Autodesk Inventor part; units mm, degrees
ref_plane "YZ Plane" through (0, 0, 0) normal (1, 0, 0) x (0, 1, 0)
ref_plane "XZ Plane" through (0, 0, 0) normal (0, 1, 0) x (-1, 0, 0)
ref_plane "XY Plane" through (0, 0, 0) normal (0, 0, 1) x (1, 0, 0)
sketch "Sketch1" plane through (0, 0, 0) normal (0, 1, 0) x (-1, 0, 0)
  circle A0 centre (0, 0) radius 8.575
  dimension "d0" = 17.15
extrude "Extrusion1" add sketch "Sketch1" along normal blind 75.5
sketch "Sketch2" plane through (0, 75.5, 0) normal (0, 1, 0) x (1, 0, 0)
  circle A0 centre (0, 0) radius 8.85
  dimension "d3" = 17.7
extrude "Extrusion2" add sketch "Sketch2" against normal blind 9.6
sketch "Sketch3" plane through (0, 75.5, 0) normal (0, 1, 0) x (1, 0, 0)
  line L0 (-3.3083, -9.5957) -> (-10.4021, -7.15)
  arc A0 (-10.4021, 7.15) -> (-10.4021, -7.15) centre (-7.937, 0) ccw
  line L1 (-10.4021, 7.15) -> (-3.3083, 9.5957)
  arc A1 (3.3083, 9.5957) -> (-3.3083, 9.5957) centre (0, 0) ccw
  line L2 (3.3083, 9.5957) -> (10.4021, 7.15)
  arc A2 (10.4021, -7.15) -> (10.4021, 7.15) centre (7.937, 0) ccw
  line L3 (10.4021, -7.15) -> (3.3083, -9.5957)
  arc A3 (-3.3083, -9.5957) -> (3.3083, -9.5957) centre (0, 0) ccw
  line L4 (0, -10.15) -> (0, 10.15) construction
  line L5 (-15.5, 0) -> (15.5, 0) construction
  dimension "d6" = 20.3
  dimension "d7" = 31
  dimension "d8" = 14.3
extrude "Extrusion3" add sketch "Sketch3" against normal blind 2
sketch "Sketch4" plane through (0, 75.5, 0) normal (0, 1, 0) x (1, 0, 0)
  circle A0 centre (0, 0) radius 7.875
  dimension "d11" = 15.75
extrude "Extrusion4" cut sketch "Sketch4" against normal blind 74.5
sketch "Sketch5" plane through (0, 0, 0) normal (0, -1, 0) x (1, 0, 0)
  circle A0 centre (0, -5.075) radius 2.5
  point P0 (0, 0)
  dimension "d14" = 5
ref_plane "Work Plane1" through (0, -10, 0) normal (0, -1, 0) x (1, 0, 0)
sketch "Sketch6" plane through (0, -10, 0) normal (0, -1, 0) x (1, 0, 0)
  circle A0 centre (0, -5.075) radius 2
  point P0 (0, 0)
  dimension "d18" = 4
loft "Loft1" add profiles "Sketch5", "Sketch6"
sketch "Sketch7" plane through (0, -10, -5.075) normal (0, -1, 0) x (1, 0, 0)
  circle A0 centre (0, 0) radius 2
  circle A1 centre (0, 0) radius 1.2
  point P0 (0, 5.075)
  dimension "d24" = 0.8
extrude "Extrusion5" cut sketch "Sketch7" against normal through all contours A1
properties part number "Syringe" material "Glass"
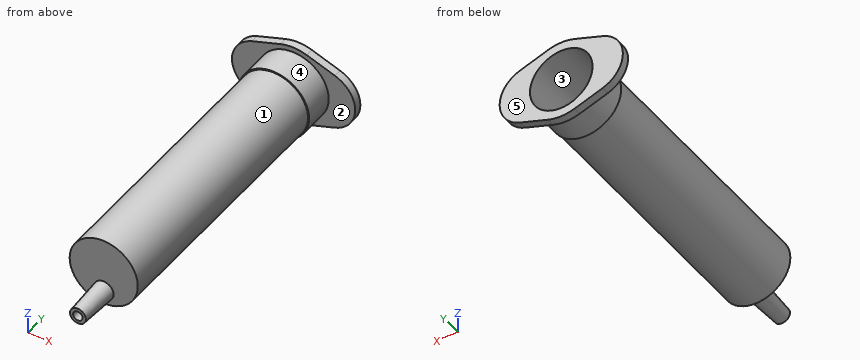
Could you check a few things on this model? Use its own coordinates, in mm. Face numbers are marked on the shaded views. A direction names the side the tool comes from. Round coordinates to 2 decimals unless told otherwise and drop trailing zeros. Loops run counter-clockwise (first coordinate to the right, second up) from the corner with the lowest first, then second, coordinate; pieces in that order, holes last. Notation, with made-up numbers: (18, 81.25) - (40, 81.25) arc R24 ccw to (40, 119.25) - close; hole circle Ø1 at (-20, 80). An arc over 180 degrees is marked (long way). Write item = value, one per line.
1) I need wall thicknesses on line 1 along X through (y, z) = (18, -0.25); line 2 along Z through (x, y) = (0, 45) (3 decimals); line 3 along Y through (x, z) = (0, -8.5). Which ranges of each line are inside material? Lowest first, please. Write a range as from..to.
Computed:
line_1 = -8.57..-7.87, 7.87..8.57
line_2 = -8.575..-7.875, 7.875..8.575
line_3 = 0..75.5
2) If we mould it in two halves opening along Z, with no side actions, what happens to the marked faces 1, 2 and 3? For each: pulls with the +Z half, pulls with the -Z half, needs draft (parallel to the pull), parting line crosses it, or undercut.
Computed:
face_1 = parting line crosses it
face_2 = needs draft
face_3 = undercut
3) I'm going to push flat-ended pins straight in: P1, Ø8, axis at x = 11, z = 4.5, coming from the -Y side; P2, Ø2, axis at y = 15, z = 6, coming from the -X side; P3, Ø9.5, axis at x = 0, z = 0, coming from the +Y side. Where does each tip first touch, or does it pass through?
Computed:
P1 = 0
P2 = -6.97
P3 = 1
4) Imagine slicing it at C-C (y = 51). Please give me the cut outline in (x, z) (3 decimals).
Computed:
outline = circle Ø17.15 at (0, 0); hole circle Ø15.75 at (0, 0)
5) On a 3-axis mill with a long thin cutter (end or side, diameter ignored), from which of +Z, -Z, +X, -X, +Y, -Y can I reach the whole of each face in a straight line? I mean the marked faces 4 and 5. Say none if no direction works.
Computed:
face_4 = -Y
face_5 = +Z, -Z, +X, -X, +Y
6) Imagine slicing it at A-A (x = 0). Please give me the cut outline in (y, z) (3 decimals), and give its area (3 significant figures).
Computed:
outline = (-10, -7.075) - (0, -7.575) - (0, -8.575) - (65.9, -8.575) - (65.9, -8.85) - (73.5, -8.85) - (73.5, -10.15) - (75.5, -10.15) - (75.5, -7.875) - (1, -7.875) - (1, -6.275) - (-10, -6.275) - close; (-10, -3.875) - (1, -3.875) - (1, 7.875) - (75.5, 7.875) - (75.5, 10.15) - (73.5, 10.15) - (73.5, 8.85) - (65.9, 8.85) - (65.9, 8.575) - (0, 8.575) - (0, -2.575) - (-10, -3.075) - close
area = 151 mm2
7) Imagine slicing it at D-D (x = 12.5). Please give me the cut outline in (y, z), and give its area (3 significant figures).
Computed:
outline = (73.5, -6.03) - (75.5, -6.03) - (75.5, 6.03) - (73.5, 6.03) - close
area = 24.1 mm2
8) Imagine slicing it at B-B (z = 0). Please give me the cut outline in (x, y) (3 decimals), and give its area (3 significant figures).
Computed:
outline = (-15.5, 73.5) - (-8.85, 73.5) - (-8.85, 65.9) - (-8.575, 65.9) - (-8.575, 0) - (8.575, 0) - (8.575, 65.9) - (8.85, 65.9) - (8.85, 73.5) - (15.5, 73.5) - (15.5, 75.5) - (7.875, 75.5) - (7.875, 1) - (-7.875, 1) - (-7.875, 75.5) - (-15.5, 75.5) - close
area = 153 mm2
